Model file for the job. Use its own axes, mm. A direction names the side the tool comes from. Round coordinates to 2 decimals unless told otherwise and drop trailing zeros. Write each loop counter-clockwise with the first axis right and the second up, starting at its lowest first coordinate (ties: lowest second). Pieces come first, ordered by that corner, then holes. Notation, with made-up numbers: (68.25, 29.5) - (91.25, 29.5) arc R25 cw to (91.25, 62.5) - close; hole circle Ø11 at (81.25, 7.5). An arc over 180 degrees is marked (long way). One line per item, written item: value.
from build123d import *

# Parameters (mm, degrees)
SKETCH1_W              = 18.2626
SKETCH1_H              = 32.9184
MAIN_BODY_DEPTH        = 13.97
SKETCH2_W              = 45.72
SKETCH2_H              = 6.223
BOTTOM_BODY_DEPTH      = 13.97
SKETCH3_R              = 4.0005
CENTER_HOLE_DEPTH      = 1
CENTER_HOLE_DEPTH_BACK = 14.97
SKETCH4_W              = 1.524
SKETCH4_H              = 24.062462206
CENTER_CUT_DEPTH       = 14.97
SKETCH5_R              = 3.7719
SIDE_HOLE_DEPTH        = 32.9913
F_5_0MM_DOWEL_HOLE1_D  = 5


with BuildPart() as part:
    # Sketch1 → Main Body] (new body)
    with BuildSketch(Plane.XY):
        Rectangle(SKETCH1_W, SKETCH1_H)
    extrude(amount=MAIN_BODY_DEPTH)

    # Sketch2 → Bottom Body (add)
    with BuildSketch(Plane.XY.offset(13.97)):
        with Locations((0, -13.3477)):
            Rectangle(SKETCH2_W, SKETCH2_H)
    extrude(amount=-BOTTOM_BODY_DEPTH)

    # Sketch3 → Center Hole (cut, two sides)
    with BuildSketch(Plane.XY.offset(13.97)) as center_hole_sk:
        with Locations((0, 3.7592)):
            Circle(SKETCH3_R)
    extrude(amount=CENTER_HOLE_DEPTH, mode=Mode.SUBTRACT)
    extrude(center_hole_sk.sketch, amount=-CENTER_HOLE_DEPTH_BACK, mode=Mode.SUBTRACT)

    # Sketch4 → Center Cut (cut, through all)
    with BuildSketch(Plane.XY.offset(13.97)):
        with Locations((0, 16.4592)):
            Rectangle(SKETCH4_W, SKETCH4_H)
    extrude(amount=-CENTER_CUT_DEPTH, mode=Mode.SUBTRACT)

    # Sketch5 → Side Hole (cut, through all)
    with BuildSketch(Plane(origin=(9.1313, 0, 0), x_dir=(0, 0, -1), z_dir=(1, 0, 0))):
        with Locations((-7.196820587, 12.3952)):
            Circle(SKETCH5_R)
    extrude(amount=-SIDE_HOLE_DEPTH, mode=Mode.SUBTRACT)

    # Ø5.0mm Dowel Hole1 (through all)
    with Locations(Plane(origin=(0, -10.2362, 0), x_dir=(1, 0, 0), z_dir=(0, 1, 0))):
        with Locations((15.24, -7.62)):
            f_5_0mm_dowel_hole1 = Hole(F_5_0MM_DOWEL_HOLE1_D / 2)

    # Mirror1: Ø5.0mm Dowel Hole1 across plane
    add(f_5_0mm_dowel_hole1.mirror(Plane(origin=(0, 0, 0), x_dir=(0, 0, 1), z_dir=(1, 0, 0))), mode=Mode.SUBTRACT)


solid = part.part
1. Tool access for faces 1 (the face through (0, -16.459, 7)), 2 (the face through (-18, -10.236, 6)), 3 (the face through (17.4, -10.236, 5.5)), 4 (the face through (0.762, 10, 4)), 5 (the face through (5, 16.459, 7)): list every direction of +Z, -Z, +X, -X, +Y, -Y with a clear straight run to the whole face (end or side of a thin tool).
Report:
face 1: +Z, -Z, +X, -X, -Y
face 2: +Z, -Z, -X, +Y
face 3: +Z, -Z, +X, +Y
face 4: +Z, -Z, +Y
face 5: +Z, -Z, +X, -X, +Y
2. Band-saw the part on C-C on x = -16. Write the cut outline in (y, z), plus the area to 3 significant figures.
Report:
outline: (-16.46, 0) - (-10.24, 0) - (-10.24, 5.24) - (-16.46, 5.24) - close; (-16.46, 10) - (-10.24, 10) - (-10.24, 13.97) - (-16.46, 13.97) - close
area: 57.3 mm²
3. Band-saw the part on D-D on y = -14. Write the cut outline in (x, z), plus the area to 3 significant figures.
Report:
outline: (-22.86, 0) - (22.86, 0) - (22.86, 13.97) - (-22.86, 13.97) - close; hole circle Ø5 at (-15.24, 7.62); hole circle Ø5 at (15.24, 7.62)
area: 599 mm²
4. Mould opens along X. For faces 6 (the face through (9.131, 0, 7)), 7 (the face through (-9.131, 0, 7)), 8 (the face through (17.224, -13.391, 9.141)), 9 (the face through (-17.224, -13.391, 9.141)) say: released by +X, released by -X, zero draft, split by the parting line, or undercut.
Report:
face 6: released by +X
face 7: released by -X
face 8: undercut
face 9: undercut
5. Drop flat-ended pins along their axis: pin 1 (4 mm diameter, centred on x = -17.5, z = 10.5, fed in from +Y); pin 2 (2 mm diameter, centred on y = 4, z = 2.5, fed in from +X); pin 3 (1.5 mm diameter, centred on y = 4.5, z = 5, fed in from -X). Give the stop position or say it passes through.
Report:
pin 1: y = -10.24
pin 2: x = 9.13
pin 3: x = -9.13
6. Band-saw the part on B-B on z = 1.5. Write the cut outline in (x, y), plus the area to 3 significant figures.
Report:
outline: (-22.86, -16.46) - (22.86, -16.46) - (22.86, -10.24) - (9.13, -10.24) - (9.13, 16.46) - (0.76, 16.46) - (0.76, 7.69) arc R4 cw (long way) to (-0.76, 7.69) - (-0.76, 16.46) - (-9.13, 16.46) - (-9.13, -10.24) - (-22.86, -10.24) - close
area: 708 mm²
7. Band-saw the part on A-A on x = 3. Write the cut outline in (y, z).
Report:
outline: (-16.46, 0) - (1.11, 0) - (1.11, 13.97) - (-16.46, 13.97) - close; (6.41, 0) - (16.46, 0) - (16.46, 13.97) - (6.41, 13.97) - close; hole circle Ø7.54 at (12.4, 7.2)
8. Wall check: probe 1 along Z at (x, y) = (15, -12.5); probe 2 along Y at (x, z) = (-12.5, 12.5); probe 3 along Y at (x, z) = (-2.5, 9.75). Give the ranges that are in metal, low to high. Write a range as [from, to].
Report:
probe 1: [0, 5.13], [10.11, 13.97]
probe 2: [-16.46, -10.24]
probe 3: [-16.46, 0.64], [6.88, 9.62], [15.17, 16.46]
